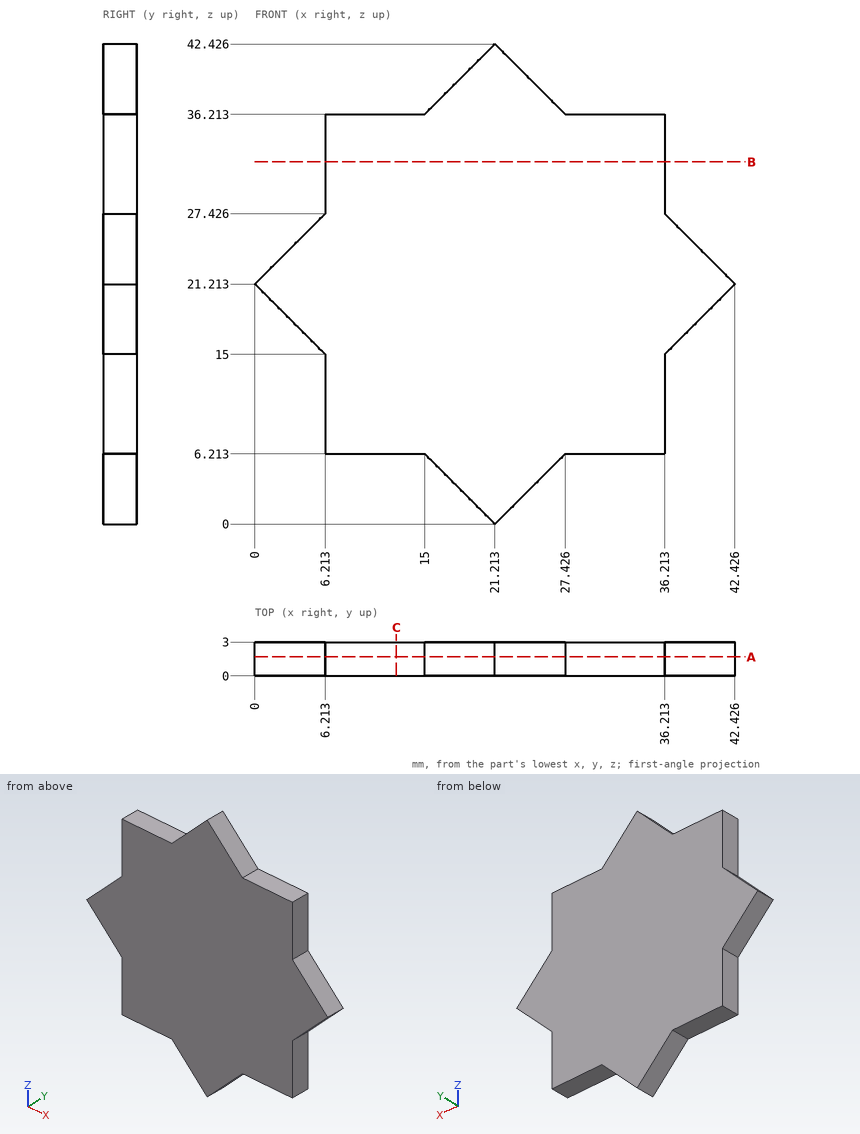
Check sheet for the drawn part. Datum: minimum x, y, z corner. Units: mm. Coordinates: 2 decimals unless noted, no trailing zeros. Write each loop counter-clockwise with the first axis right and the second up, starting at its lowest first coordinate (ties: lowest second). Pieces come first, ordered by that corner, then holes. Notation, with made-up numbers: M 44.25,41.25 L 89.25,41.25 A5 ccw 89.25,48.25 Z; hole C 51,-21 d4. An arc over 180 degrees is marked long. One line per item, written item: value.
Item 1: Section check B-B, the plane z = 32. Record the boundary of the cut face in (x, y).
Check sheet entries:
outline: M 6.21,0 L 36.21,0 L 36.21,3 L 6.21,3 Z
Item 2: Section check A-A, the plane y = 1.7. Record the boundary of the cut face in (x, z), plus the area to 3 significant figures.
Check sheet entries:
outline: M 0,21.21 L 6.21,15 L 6.21,6.21 L 15,6.21 L 21.21,0 L 27.43,6.21 L 36.21,6.21 L 36.21,15 L 42.43,21.21 L 36.21,27.43 L 36.21,36.21 L 27.43,36.21 L 21.21,42.43 L 15,36.21 L 6.21,36.21 L 6.21,27.43 Z
area: 1,050 mm^2
Item 3: Scan lines: line 1 along X through (y, z) = (0.25, 29.5); line 2 along X through (y, z) = (1.8, 4.5) (1 decimal). Record each from-to range of solid material in increasing order.
Check sheet entries:
line 1: x = 6.21 to 36.21
line 2: x = 16.7 to 25.7
Item 4: Gauge pin test, flat ends, axial feed: pin 1 Ø5 at (x, z) = (10.5, 19.5) entering from -Y; pin 2 Ø0.9 at (x, y) = (9, 2) entering from +Z; pin 3 Ø0.9 at (y, z) = (1.5, 9.5) entering from +X; pin 4 Ø0.9 at (y, z) = (1, 33) entering from -X. Record the tip position at first contact, or that the pin passes through.
Check sheet entries:
pin 1: stops at y = 0
pin 2: stops at z = 36.21
pin 3: stops at x = 36.21
pin 4: stops at x = 6.21
Item 5: Section check C-C, the plane x = 12.5. Record the boundary of the cut face in (y, z).
Check sheet entries:
outline: M 0,6.21 L 3,6.21 L 3,36.21 L 0,36.21 Z
